Autodesk Inventor part; units mm, degrees
ref_plane "YZ Plane" through (0, 0, 0) normal (1, 0, 0) x (0, 1, 0)
ref_plane "XZ Plane" through (0, 0, 0) normal (0, 1, 0) x (-1, 0, 0)
ref_plane "XY Plane" through (0, 0, 0) normal (0, 0, 1) x (1, 0, 0)
sketch "Sketch1" plane through (0, 0, 0) normal (1, 0, 0) x (0, 1, 0)
  circle A0 centre (-6.9088, 6.9088) radius 1.778
  circle A1 centre (6.9088, 6.9088) radius 1.778
  circle A2 centre (-6.9088, -6.9088) radius 1.778
  circle A3 centre (6.9088, -7.1628) radius 1.778
  line L0 (-10.0838, 10.0838) -> (10.0838, 10.0838)
  line L1 (10.0838, 10.0838) -> (10.0838, -10.0838)
  line L2 (10.0838, -10.0838) -> (-10.0838, -10.0838)
  line L3 (-10.0838, -10.0838) -> (-10.0838, 10.0838)
  point P0 (0, 0)
  dimension "d0" = 6.9088
  dimension "d1" = 6.9088
  dimension "d2" = 13.8176
  dimension "d3" = 13.8176
  dimension "d4" = 3.556
  dimension "d5" = 3.556
  dimension "d6" = 3.556
  dimension "d7" = 3.556
  dimension "d8" = 3.175
  dimension "d9" = 3.175
  dimension "d10" = 3.175
  dimension "d11" = 3.175
extrude "Extrusion1" add sketch "Sketch1" along normal blind 9.525
sketch "Sketch2" plane through (0, 10.0838, 10.0838) normal (0, 1, 0) x (1, 0, 0)
  circle A0 centre (4.7625, 9.9568) radius 3.175
  line L0 (0, 0) -> (0, 20.1676)
  line L1 (0, 20.1676) -> (9.525, 20.1676)
  point P0 (0, 10.0838)
  dimension "d14" = 6.35
  dimension "d17" = 4.7625
  dimension "d18" = 10.2108
extrude "Extrusion2" cut sketch "Sketch2" against normal blind 38.1
sketch "Sketch3" plane through (9.525, 0, 0) normal (1, 0, 0) x (0, 0, -1)
  circle A0 centre (0, 0) radius 1.7526
  dimension "d19" = 3.5052
extrude "Extrusion3" cut sketch "Sketch3" against normal blind 4.7625
properties part number "Tube Bracket"
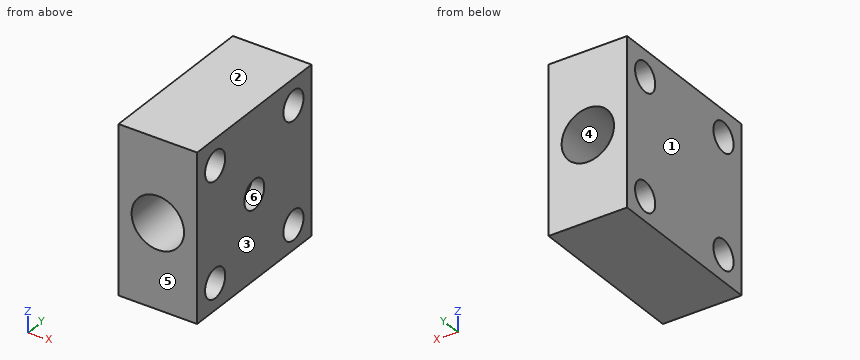
Geometry check sheet. Reference: the model listing, model coordinates, mm. Face numbers are marked on the shaded views. A direction names the side the tool comes from. Give positions to 0.01 mm unless a question says otherwise; leave off trailing zeros. Loops run counter-clockwise (first coordinate to the right, second up) from the corner with the lowest first, then second, coordinate; pieces in that order, holes last. Notation, with made-up numbers: (35.25, -31) - (84.25, -31) arc R31 ccw to (84.25, 5) - close; hole circle Ø8 at (-1, 0.5). An arc over 180 degrees is marked (long way). Use CSV: the item, a comma, the result in double quotes. Start each with the question number.
Q1. Release check for a two-part mould opening along X. For the marked faces 1, 2, 3 and 4 record: +X half, -X half, draft (parallel to the pull), parting line (faces both ways), or undercut.
Q2. Scan lines: probe 1 along Z at (x, y) = (6.75, 5.5); probe 2 along Z at (x, y) = (2, -7); probe 3 along Y at (x, z) = (8.25, 7.75). Record each from-to range of solid material in increasing order. Write a range as from..to.
Q3. Section check A-A, the plane x = 4.5. Record the cut outline in (y, z), and give its area (3 significant figures).
Q4. Section check C-C, the plane z = -0.75. Record the cut outline in (x, y) (3 decimals).
Q5. Section check D-D, the plane z = 2.25. Record the cut outline in (x, y) (3 decimals).
Q6. Section check B-B, the plane y = -6.75. Count the separate pieces of the cut face and the enclosed holes in it, and give its area (3 significant figures).
Q7. Access from +Z, -Z, +X, -X, +Y, -Y to the whole of each face (thin tool, end or side, straight path). Record for the marked faces 5 and 6.
Findings below:
1,face 1,"-X half"
1,face 2,"draft"
1,face 3,"+X half"
1,face 4,"undercut"
2,probe 1,"z = -10.08..-8.25, -6.08..-2.35, 2.6..5.82, 7.99..10.08"
2,probe 2,"z = -10.08..-8.68, -5.13..-1.44, 1.69..5.13, 8.68..10.08"
2,probe 3,"y = -10.08..-8.48, -5.34..5.34, 8.48..10.08"
3,outline,"(-10.08, -10.08) - (10.08, -10.08) - (10.08, -3.04) - (-10.08, -3.04) - close; (-10.08, 3.29) - (10.08, 3.29) - (10.08, 10.08) - (-10.08, 10.08) - close; hole circle Ø3.56 at (-6.91, -6.91); hole circle Ø3.56 at (-6.91, 6.91); hole circle Ø3.56 at (6.91, -7.16); hole circle Ø3.56 at (6.91, 6.91)"
3,area,"239 mm^2"
4,outline,"(0, -10.084) - (1.711, -10.084) - (1.711, 10.084) - (0, 10.084) - close; (7.814, -10.084) - (9.525, -10.084) - (9.525, -1.584) - (7.814, -1.584) - close; (7.814, 1.584) - (9.525, 1.584) - (9.525, 10.084) - (7.814, 10.084) - close"
5,outline,"(0, -10.084) - (2.402, -10.084) - (2.402, 10.084) - (0, 10.084) - close; (7.123, -10.084) - (9.525, -10.084) - (9.525, 10.084) - (7.123, 10.084) - close"
6,separate pieces,"3"
6,enclosed holes,"1"
6,area,"93.0 mm^2"
7,face 5,"+Z, -Z, +X, -X, -Y"
7,face 6,"+X"
